Source: CAD feature listing. Evaluate the final solid. Frame: model axes, mm. Give positions to 0.01 mm unless a question says otherwise; leave off trailing zeros. Order: outer loops, then holes, each group sorted by start corner. A loop starts at its lowest first (then second) coordinate and runs counter-clockwise, first axis right, second up. Notation, with made-up numbers: (19.5, 30) -> (76.5, 30) arc R18 cw to (76.5, 46) -> close; hole circle Ø5 at (32.25, 15). An arc over 180 degrees is marked (long way). Answer in a Markdown table with one row per item.
```python
from build123d import *

# Parameters (mm, degrees)
BOSS_EXTRUDE1_DEPTH     = 2.54
F_8_CLEARANCE_HOLE1_D   = 4.4958
F_1_4_CLEARANCE_HOLE1_D = 6.7564
SKETCH6_R               = 9.525
CUT_EXTRUDE1_DEPTH      = 192.999314468


with BuildPart() as part:
    # Sketch1 → Boss-Extrude1 (new body)
    with BuildSketch(Plane(origin=(0, 0, 0), x_dir=(1, 0, 0), z_dir=(0, 1, 0))):
        with BuildLine():
            Line((0, 50.726050891), (0, 3.175))
            ThreePointArc((0, 3.175), (0.92993597, 0.92993597), (3.175, 0))
            Line((3.175, 0), (173.0375, 0))
            ThreePointArc((173.0375, 0), (175.28256403, 0.92993597), (176.2125, 3.175))
            Line((176.2125, 3.175), (176.2125, 73.025))
            ThreePointArc((176.2125, 73.025), (175.28256403, 75.27006403), (173.0375, 76.2))
            Line((173.0375, 76.2), (47.753083613, 76.2))
            ThreePointArc((47.753083613, 76.2), (41.179079868, 75.334515988), (35.053083613, 72.797045256))
            Line((35.053083613, 72.797045256), (1.5875, 53.475681548))
            ThreePointArc((1.5875, 53.475681548), (0.425369343, 52.313550891), (0, 50.726050891))
        make_face()
    extrude(amount=BOSS_EXTRUDE1_DEPTH)

    # #8 Clearance Hole1 (through all)
    with Locations(Plane(origin=(0, 2.54, 0), x_dir=(1, 0, 0), z_dir=(0, 1, 0))):
        with Locations((12.7, 12.7), (38.1, 12.7), (88.9, 12.7), (63.5, 12.7), (114.3, 12.7), (139.7, 12.7), (165.1, 12.7), (165.1, 63.5), (165.1, 38.1), (12.7, 38.1)):
            Hole(F_8_CLEARANCE_HOLE1_D / 2)

    # 1/4 Clearance Hole1 (through all)
    with Locations(Plane(origin=(0, 2.54, 0), x_dir=(1, 0, 0), z_dir=(0, 1, 0))):
        with Locations((37.25, 30.9), (37.25, 64.9), (71.25, 64.9), (71.25, 30.9)):
            Hole(F_1_4_CLEARANCE_HOLE1_D / 2)

    # Sketch6 → Cut-Extrude1 (cut, through all)
    with BuildSketch(Plane.XZ):
        with Locations(Location((54.25, -47.9, 0), (0, 0, 270))):
            Circle(SKETCH6_R)
        with BuildLine():
            Line((149.225, -66.675), (110.541932823, -66.675))
            ThreePointArc((110.541932823, -66.675), (105.949557162, -63.174043513), (108.108974619, -57.818343112))
            Line((108.108974619, -57.818343112), (148.379541796, -33.887504729))
            ThreePointArc((148.379541796, -33.887504729), (153.167753999, -33.842315673), (155.575, -37.981661618))
            Line((155.575, -37.981661618), (155.575, -60.325))
            ThreePointArc((155.575, -60.325), (153.715128061, -64.815128061), (149.225, -66.675))
        make_face()
        with BuildLine():
            Line((125.808067177, -22.225), (87.125, -22.225))
            ThreePointArc((87.125, -22.225), (82.634871939, -24.084871939), (80.775, -28.575))
            Line((80.775, -28.575), (80.775, -50.918338382))
            ThreePointArc((80.775, -50.918338382), (83.182246001, -55.057684327), (87.970458204, -55.012495271))
            Line((87.970458204, -55.012495271), (128.241025381, -31.081656888))
            ThreePointArc((128.241025381, -31.081656888), (130.400442838, -25.725956487), (125.808067177, -22.225))
        make_face()
    extrude(amount=-CUT_EXTRUDE1_DEPTH, mode=Mode.SUBTRACT)


solid = part.part
```
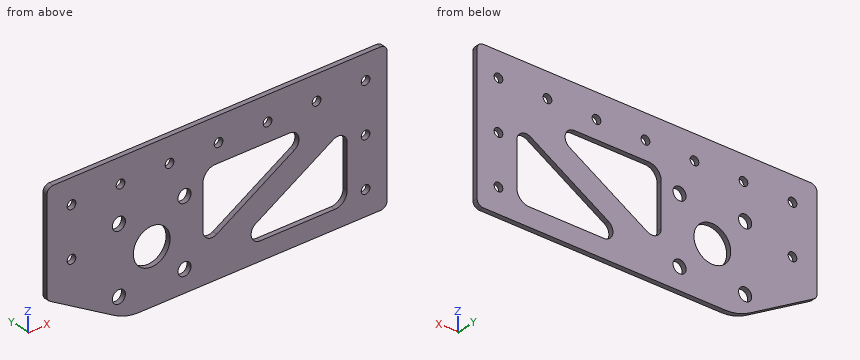
(1) Section query D-D (y = 1.5). Give the number of separate pieces and of enclosed holes in the cut face, plus the area to 3 significant figures.
A:
| item | result |
|---|---|
| separate pieces | 1 |
| enclosed holes | 17 |
| area | 10,200 mm^2 |
(2) Section query A-A (x = 165.1). Return the cut outline in (y, z).
A:
| item | result |
|---|---|
| outline | (0, -76.2) -> (2.54, -76.2) -> (2.54, -65.75) -> (0, -65.75) -> close; (0, -61.25) -> (2.54, -61.25) -> (2.54, -40.35) -> (0, -40.35) -> close; (0, -35.85) -> (2.54, -35.85) -> (2.54, -14.95) -> (0, -14.95) -> close; (0, -10.45) -> (2.54, -10.45) -> (2.54, 0) -> (0, 0) -> close |
(3) Section query B-B (x = 71.25). Return the cut outline in (y, z), plus the area to 3 significant figures.
A:
| item | result |
|---|---|
| outline | (0, -76.2) -> (2.54, -76.2) -> (2.54, -68.28) -> (0, -68.28) -> close; (0, -61.52) -> (2.54, -61.52) -> (2.54, -34.28) -> (0, -34.28) -> close; (0, -27.52) -> (2.54, -27.52) -> (2.54, 0) -> (0, 0) -> close |
| area | 159 mm^2 |
(4) Section query C-C (z = -47.9). Return the cut outline in (x, y) (1 decimal), plus the area to 3 significant figures.
A:
| item | result |
|---|---|
| outline | (0, 0) -> (44.7, 0) -> (44.7, 2.5) -> (0, 2.5) -> close; (63.8, 0) -> (80.8, 0) -> (80.8, 2.5) -> (63.8, 2.5) -> close; (99.9, 0) -> (124.8, 0) -> (124.8, 2.5) -> (99.9, 2.5) -> close; (155.6, 0) -> (176.2, 0) -> (176.2, 2.5) -> (155.6, 2.5) -> close |
| area | 272 mm^2 |
(5) Ray query, probe 1 along Z at (x, y) = (38.1, 0.9); probe 2 along X at (y, z) = (0.4, -29.5) (1 decimal); probe 3 along X at (y, z) = (2.1, -48.5) (1 decimal). Return the intervals inside material, ascending.
A:
| item | result |
|---|---|
| probe 1 | z = -74.29 to -68.17, -61.63 to -34.17, -27.63 to -14.95, -10.45 to 0 |
| probe 2 | x = 0 to 34.2, 40.3 to 68.2, 74.3 to 80.8, 129.9 to 176.2 |
| probe 3 | x = 0 to 44.7, 63.8 to 80.8, 98.9 to 123.8, 155.6 to 176.2 |
(6) First-contact query: pin 1 Ø5.5 at (x, z) = (37.25, -64.9) entering from -Y; pin 2 Ø6 at (x, z) = (88.9, -12.7) entering from +Y. Flat tips, straight axial feed; report the tip coordinate or a pass-through.
A:
| item | result |
|---|---|
| pin 1 | passes through |
| pin 2 | stops at y = 2.54 |
